Geometry check sheet. Reference: the model listing, model coordinates, mm. Face numbers are marked on the shaded views. A direction names the side the tool comes from. Give positions to 0.01 mm unless a question says otherwise; leave off trailing zeros. Order: outer loops, then holes, each group sorted by start corner. A loop starts at its lowest first (then second) coordinate and runs counter-clockwise, first axis right, second up. Notation, with made-up numbers: (-35, 47) - (-14, 47) arc R18 ccw to (-14, 58) - close; hole circle Ø6 at (52, 7). An arc over 180 degrees is marked (long way). Put each result on its own line as item: value. Start each with the question number.
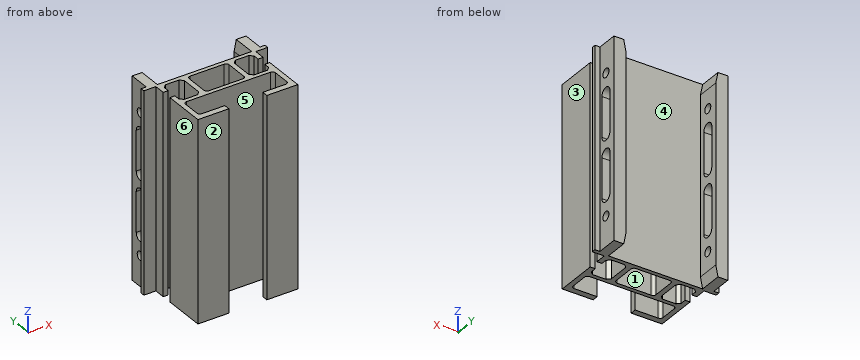
```python
from build123d import *
from OCP.BRepFilletAPI import BRepFilletAPI_MakeChamfer

# Parameters (mm, degrees)
SCHIZZO1_W                   = 20
SCHIZZO1_H                   = 14
ESTRUSIONE_ESTRUSIONE1_DEPTH = 100
SMUSSO1_SIZE                 = 1.6
RACCORDO1_R                  = 1.5
SMUSSO2_SIZE                 = 5.5
SMUSSO2_SIZE2                = 1.1
SMUSSO3_SIZE                 = 5.5
SMUSSO3_SIZE2                = 1.1
FORO_PER_VITE_M4_1_D         = 4.5
FORO_PER_VITE_M4_1_DEPTH     = 188
FORO_PER_VITE_M4_1_TIP       = 1.351936393
TAGLIO_ESTRUSIONE1_DEPTH     = 81


with BuildPart() as part:
    # Schizzo1 → Estrusione-Estrusione1 (new body)
    with BuildSketch(Plane.XY):
        Polygon((0, 0), (15.5, 0), (15.5, 21), (13, 21), (13, 16.5), (3, 16.5), (3, 30.5), (13, 30.5), (13, 26), (15.5, 26), (15.5, 31.5), (21.5, 31.5), (21.5, 33.5), (19, 33.5), (19, 44), (13, 44), (13, 32.5), (-32, 32.5), (-32, 44), (-38, 44), (-38, 33.5), (-40.5, 33.5), (-40.5, 31.5), (-34.5, 31.5), (-34.5, 26), (-32, 26), (-32, 30.5), (-22, 30.5), (-22, 16.5), (-32, 16.5), (-32, 21), (-34.5, 21), (-34.5, 0), (-19, 0), (-19, 3), (-32, 3), (-32, 14.5), (13, 14.5), (13, 3), (0, 3), align=None)
        with Locations((-9.5, 23.5)):
            Rectangle(SCHIZZO1_W, SCHIZZO1_H, mode=Mode.SUBTRACT)
    extrude(amount=ESTRUSIONE_ESTRUSIONE1_DEPTH)

    # Smusso1
    smusso1_edges = [part.edges().sort_by_distance(p)[0] for p in [
        (-32, 16.5, 50),
        (-22, 16.5, 50),
        (-22, 30.5, 50),
        (-32, 30.5, 50),
        (13, 30.5, 50),
        (3, 30.5, 50),
        (3, 16.5, 50),
        (13, 16.5, 50),
    ]]
    chamfer(smusso1_edges, length=SMUSSO1_SIZE)

    # Raccordo1
    raccordo1_edges = [part.edges().sort_by_distance(p)[0] for p in [
        (13, 3, 50),
        (13, 14.5, 50),
        (-32, 14.5, 50),
        (-32, 3, 50),
        (-19.5, 30.5, 50),
        (-19.5, 16.5, 50),
        (0.5, 16.5, 50),
        (0.5, 30.5, 50),
    ]]
    fillet(raccordo1_edges, radius=RACCORDO1_R)

    # Smusso2: one chamfer whose edges measure the first distance from different faces: ONE call of the kernel's chamfer builder (chamfer() names one face for all edges)
    smusso2_edges_1 = [part.edges().sort_by_distance(p)[0] for p in [
        (13, 38.25, 100),
    ]]
    smusso2_side_1 = [part.faces().sort_by_distance(p)[0] for p in [
        (13, 38.25, 50),
    ]]
    smusso2_edges_2 = [part.edges().sort_by_distance(p)[0] for p in [
        (-32, 38.25, 100),
    ]]
    smusso2_side_2 = [part.faces().sort_by_distance(p)[0] for p in [
        (-32, 38.25, 50),
    ]]
    smusso2 = BRepFilletAPI_MakeChamfer(part.part.solid().wrapped)
    for e in smusso2_edges_1:
        smusso2.Add(SMUSSO2_SIZE, SMUSSO2_SIZE2, e.wrapped, smusso2_side_1[0].wrapped)  # the first distance lies on this face
    for e in smusso2_edges_2:
        smusso2.Add(SMUSSO2_SIZE, SMUSSO2_SIZE2, e.wrapped, smusso2_side_2[0].wrapped)  # the first distance lies on this face
    add(Compound.cast(smusso2.Shape()), mode=Mode.REPLACE)

    # Smusso3: one chamfer whose edges measure the first distance from different faces: ONE call of the kernel's chamfer builder (chamfer() names one face for all edges)
    smusso3_edges_1 = [part.edges().sort_by_distance(p)[0] for p in [
        (-32, 38.25, 0),
    ]]
    smusso3_side_1 = [part.faces().sort_by_distance(p)[0] for p in [
        (-32, 38.25, 47.25),
    ]]
    smusso3_edges_2 = [part.edges().sort_by_distance(p)[0] for p in [
        (13, 38.25, 0),
    ]]
    smusso3_side_2 = [part.faces().sort_by_distance(p)[0] for p in [
        (13, 38.25, 47.25),
    ]]
    smusso3 = BRepFilletAPI_MakeChamfer(part.part.solid().wrapped)
    for e in smusso3_edges_1:
        smusso3.Add(SMUSSO3_SIZE, SMUSSO3_SIZE2, e.wrapped, smusso3_side_1[0].wrapped)  # the first distance lies on this face
    for e in smusso3_edges_2:
        smusso3.Add(SMUSSO3_SIZE, SMUSSO3_SIZE2, e.wrapped, smusso3_side_2[0].wrapped)  # the first distance lies on this face
    add(Compound.cast(smusso3.Shape()), mode=Mode.REPLACE)

    # Foro per Vite M4-1
    with Locations(Plane(origin=(19, 0, 0), x_dir=(0, 0, -1), z_dir=(1, 0, 0))):
        with Locations((-85, 38), (-15, 38)):
            Hole(FORO_PER_VITE_M4_1_D / 2, depth=FORO_PER_VITE_M4_1_DEPTH)
            with Locations((0, 0, -(FORO_PER_VITE_M4_1_DEPTH + FORO_PER_VITE_M4_1_TIP / 2))):  # 118° drill point
                Cone(0, FORO_PER_VITE_M4_1_D / 2, FORO_PER_VITE_M4_1_TIP, mode=Mode.SUBTRACT)

    # Schizzo4 → Taglio-Estrusione1 (cut)
    with BuildSketch(Plane(origin=(19, 0, 0), x_dir=(0, 0, -1), z_dir=(1, 0, 0))):
        with BuildLine():
            Line((-75, 41), (-55, 41))
            ThreePointArc((-55, 41), (-52, 38), (-55, 35))
            Line((-55, 35), (-75, 35))
            ThreePointArc((-75, 35), (-78, 38), (-75, 41))
        make_face()
        with BuildLine():
            Line((-45, 41), (-25, 41))
            ThreePointArc((-25, 41), (-22, 38), (-25, 35))
            Line((-25, 35), (-45, 35))
            ThreePointArc((-45, 35), (-48, 38), (-45, 41))
        make_face()
    extrude(amount=-TAGLIO_ESTRUSIONE1_DEPTH, mode=Mode.SUBTRACT)


solid = part.part
```
Item 1: Gauge pin test, flat ends, axial feed: pin 1 Ø2.5 at (y, z) = (10.5, 57.5) entering from -X; pin 2 Ø1.8 at (x, z) = (-35.5, 67) entering from -Y; pin 3 Ø6 at (y, z) = (38, 15) entering from +X; pin 4 Ø1 at (x, y) = (11.5, 37) entering from -Z. Record the tip position at first contact, or that the pin passes through.
Item 2: Thickness scan on line 1 along X through (y, z) = (18.5, 54); line 2 along Y through (x, z) = (-34.15, 15); line 3 along Y through (x, z) = (10, 94.5). Record the ranges inside material, lowest first.
Item 3: Cross-section at C-C (x = -13). Enter the section's corners in (y, z).
Item 4: Cross-section at D-D (z = 41.5). Count the separate pieces of the cut face and the enclosed holes in it, and give its area (3 significant figures).
Item 5: Cross-section at A-A (y = 9). Enter the section's corners in (x, z).
Item 6: Release check for a two-part mould opening along Y. For the marked faces 4, 5 and 6 record: +Y half, -Y half, draft (parallel to the pull), parting line (faces both ways), or undercut.
Item 7: Set-up check for the marked faces 1, 2 and 3: record each of +Z, -Z, +X, -X, +Y, -Y from which the full face is reachable in a straight line by a thin tool's end or side.
Item 8: Cross-section at B-B (x = -27.5). Enter the section's corners in (y, z).
Recorded:
1. pin 1: stops at x = -34.5
1. pin 2: stops at y = 31.5
1. pin 3: stops at x = 19
1. pin 4: passes through
2. line 1: x = -34.5 to -32, -22 to -19.5, 0.5 to 3, 13 to 15.5
2. line 2: y = 0 to 21, 26 to 35.75, 40.25 to 44
2. line 3: y = 0 to 3, 14.5 to 16.5, 30.5 to 32.5
3. outline: (14.5, 0) - (16.5, 0) - (16.5, 100) - (14.5, 100) - close; (30.5, 0) - (32.5, 0) - (32.5, 100) - (30.5, 100) - close
4. separate pieces: 3
4. enclosed holes: 1
4. area: 563 mm^2
5. outline: (-34.5, 0) - (-32, 0) - (-32, 100) - (-34.5, 100) - close; (13, 0) - (15.5, 0) - (15.5, 100) - (13, 100) - close
6. face 4: +Y half
6. face 5: undercut
6. face 6: draft
7. face 1: +Z, -Z
7. face 2: +Z, -Z, +X, -X, -Y
7. face 3: +Z, -Z, +X, -Y
8. outline: (0, 0) - (3, 0) - (3, 100) - (0, 100) - close; (14.5, 0) - (16.5, 0) - (16.5, 100) - (14.5, 100) - close; (30.5, 0) - (32.5, 0) - (32.5, 100) - (30.5, 100) - close
